```python
from build123d import *

# Parameters (mm, degrees)
ESTRUSIONE_ESTRUSIONE1_DEPTH = 80
SCHIZZO2_R                   = 55
TAGLIO_ESTRUSIONE1_DEPTH     = 50
TAGLIO_ESTRUSIONE2_REACH     = 124.066
FORO_18_0_18_1_D             = 18
FORO_FILETTATO_M22_1_D       = 19.5
FORO_FILETTATO_M22_1_DEPTH   = 60
FORO_FILETTATO_M22_1_TIP     = 5.858391036
FORO_FILETTATO_M16_1_D       = 14
FORO_FILETTATO_M16_1_DEPTH   = 35
FORO_FILETTATO_M16_1_TIP     = 4.206024333


with BuildPart() as part:
    # Schizzo1 → Estrusione-Estrusione1 (new, symmetric)
    with BuildSketch(Plane.XY):
        Polygon((-30, 60), (30, 60), (30, 30), (60, 30), (60, -30), (30, -30), (30, -60), (-30, -60), (-30, -30), (-60, -30), (-60, 30), (-30, 30), align=None)
    extrude(amount=ESTRUSIONE_ESTRUSIONE1_DEPTH, both=True)

    # Schizzo2 → Taglio-Estrusione1 (cut)
    with BuildSketch(Plane(origin=(0, 60, 0), x_dir=(1, 0, 0), z_dir=(0, 1, 0))):
        with Locations((0, -80)):
            Circle(SCHIZZO2_R)
    extrude(amount=-TAGLIO_ESTRUSIONE1_DEPTH, mode=Mode.SUBTRACT)

    # Schizzo3 → Taglio-Estrusione2 (cut, up to next)
    with BuildSketch(Plane(origin=(0, 10, 0), x_dir=(1, 0, 0), z_dir=(0, 1, 0)), mode=Mode.PRIVATE) as taglio_estrusione2_sk1:
        with BuildLine():
            Line((-23, -72), (23, -72))
            ThreePointArc((23, -72), (31, -80), (23, -88))
            Line((23, -88), (-23, -88))
            ThreePointArc((-23, -88), (-31, -80), (-23, -72))
        make_face()
    taglio_estrusione2_tool1 = extrude(taglio_estrusione2_sk1.sketch, amount=-TAGLIO_ESTRUSIONE2_REACH, mode=Mode.PRIVATE) & part.part
    add(taglio_estrusione2_tool1.solids().sort_by_distance((0, 10, 80))[0], mode=Mode.SUBTRACT)

    # Foro Ø18.0 (18)-1 (through all)
    with Locations(Plane.ZY.offset(60)):
        with Locations((-50, 0)):
            Hole(FORO_18_0_18_1_D / 2)

    # Foro filettato M22-1
    with Locations(Plane(origin=(0, 0, -80), x_dir=(-1, 0, 0), z_dir=(0, 0, -1))):
        with Locations((0, 0)):
            Hole(FORO_FILETTATO_M22_1_D / 2, depth=FORO_FILETTATO_M22_1_DEPTH)
            with Locations((0, 0, -(FORO_FILETTATO_M22_1_DEPTH + FORO_FILETTATO_M22_1_TIP / 2))):  # 118° drill point
                Cone(0, FORO_FILETTATO_M22_1_D / 2, FORO_FILETTATO_M22_1_TIP, mode=Mode.SUBTRACT)

    # Foro filettato M16-1
    with Locations(Plane.XY.offset(72)):
        with Locations((0, -5), (0, -45)):
            Hole(FORO_FILETTATO_M16_1_D / 2, depth=FORO_FILETTATO_M16_1_DEPTH)
            with Locations((0, 0, -(FORO_FILETTATO_M16_1_DEPTH + FORO_FILETTATO_M16_1_TIP / 2))):  # 118° drill point
                Cone(0, FORO_FILETTATO_M16_1_D / 2, FORO_FILETTATO_M16_1_TIP, mode=Mode.SUBTRACT)


solid = part.part
```
Read the model definition and answer for the solid it produces. Units are mm, in the model's axes. A direction names the side the tool comes from. Give positions to 0.01 mm unless a question says otherwise; leave off trailing zeros. Order: outer loops, then holes, each group sorted by start corner. A loop starts at its lowest first (then second) coordinate and runs counter-clockwise, first axis right, second up.
(1) For a pull along X with two mould halves and no side action, classify faces 1 (the cylindrical face through (32.269, -3.447, -58.314)), 2 (the flat face through (-60, 0, 1)), 3 (the flat face through (30, 45, -22)), 4 (the conical face through (-1.62, 0.51, -15.16)) as released by +X, released by -X, zero draft, split by the parting line, or undercut.
(2) Find section A-A (z = -50). Give the vertices of the cut face in (x, y).
(3) Given pin 1 (9 mm diameter, centred on x = -46, z = 0.5, fed in from -Y); pin 2 (3 mm diameter, centred on x = -39.5, z = 18.5, fed in from +Y); pin 3 (22.5 mm diameter, centred on x = 0, y = -5, fed in from +Z), each flat-ended and moving along its own axis, determine where each tip first touches the part or whether it passes through.
(4) Find section B-B (z = -33.5). Give the vertices of the cut face in (x, y).
(5) Find section D-D (z = 21). Give the vertices of the cut face in (x, y), plus the area to 3 significant figures.
(6) Straight lines are drawn through the part: L1, parallel to Y at x = 0, z = 50.5; L2, parallel to Y at x = 0, z = -66; L3, parallel to Z at x = 21, y = 0. For each, find the intervals that lie inside material, in ascending order.
(7) Find section C-C (x = 17.5). Give the vertices of the cut face in (y, z), plus the area to 3 significant figures.
(8) For faces 5 (the flat face through (-45, -30, 1)), 6 (the cylindrical face through (1.209, 29.794, 25.013)), 7 (the flat face through (-45, 30, -17)), determine the directions among +Z, -Z, +X, -X, +Y, -Y from which every point of the face is accessible in a straight line to the end or side of a thin tool.
Result sheet:
1. face 1: zero draft
1. face 2: released by -X
1. face 3: released by +X
1. face 4: undercut
2. outline: (-60, -30) - (-30, -30) - (-30, -60) - (30, -60) - (30, -30) - (60, -30) - (60, -9) - (3.75, -9) arc R9.75 cw to (-3.75, -9) - (-60, -9) - close; (-60, 9) - (-3.75, 9) arc R9.75 cw to (3.75, 9) - (60, 9) - (60, 30) - (30, 30) - (30, 60) - (-30, 60) - (-30, 30) - (-60, 30) - close
3. pin 1: stops at y = -30
3. pin 2: stops at y = 30
3. pin 3: stops at z = 72
4. outline: (-60, -30) - (-30, -30) - (-30, -60) - (30, -60) - (30, -30) - (60, -30) - (60, 30) - (30, 30) - (30, 60) - (-30, 60) - (-30, 30) - (-60, 30) - close; hole circle Ø19.5 at (0, 0)
5. outline: (-60, -30) - (-30, -30) - (-30, -60) - (30, -60) - (30, -30) - (60, -30) - (60, 30) - (30, 30) - (30, 60) - (-30, 60) - (-30, 30) - (-60, 30) - close
5. area: 10,800 mm2
6. L1: y = -60 to -52, -38 to -12, 2 to 10
6. L2: y = -60 to -9.75, 9.75 to 60
6. L3: z = -80 to -59, -41 to 72
7. outline: (-60, -80) - (60, -80) - (60, 27.86) - (10, 27.86) - (10, 72) - (-60, 72) - close; hole circle Ø18 at (0, -50)
7. area: 15,800 mm2
8. face 5: +Z, -Z, -X, -Y
8. face 6: +Z, +Y
8. face 7: +Z, -Z, -X, +Y
